```python
from build123d import *

# Parameters (mm, degrees)
F0_W     = 55
F0_H     = 14.5
F3_DEPTH = 55
F4_R     = 4
F5_DEPTH = 16.001
F7_DEPTH = 55
F4_R_2   = 6.5
F8_DEPTH = 6


with BuildPart() as f1:
    # F0 (on Front) → F1 (revolve)
    with BuildSketch(Plane.XZ):
        with Locations((-27.5, 7.25)):
            Rectangle(F0_W, F0_H)
        Polygon((0, 16), (0, 14.5), (0, 0), (25, 0), (25, 14.5), (5, 14.5), (5, 16), align=None)
    revolve(axis=Axis((-15, 0, 0), (-1, 0, 0)))

    # F2 (on face) → F3 (cut)
    with BuildSketch(Plane(origin=(-55, 0, 0), x_dir=(0, -1, 0), z_dir=(-1, 0, 0))):
        with BuildLine():
            ThreePointArc((14.5, 0), (0, 14.5), (-14.5, 0))
            Line((-14.5, 0), (14.5, 0))
        make_face()
    extrude(amount=-F3_DEPTH, mode=Mode.SUBTRACT)

    # F4 (on face) → F5 (cut, through all)
    with BuildSketch(Plane.XY):
        with Locations((-38, 0)):
            Circle(F4_R)
        with Locations((-18, 0)):
            Circle(F4_R)
    extrude(amount=-F5_DEPTH, mode=Mode.SUBTRACT)

    # F6 (on face) → F7 (cut)
    with BuildSketch(Plane(origin=(-55, 0, 0), x_dir=(0, -1, 0), z_dir=(-1, 0, 0))):
        with BuildLine():
            ThreePointArc((-5.546382, -13.3973), (0.699618, -14.483112), (6.811879, -12.800325))
            Line((6.811879, -12.800325), (6.811879, -11.710467))
            Line((6.811879, -11.710467), (-5.546382, -11.710467))
            Line((-5.546382, -11.710467), (-5.546382, -13.3973))
        make_face()
    extrude(amount=-F7_DEPTH, mode=Mode.SUBTRACT)

    # F4 (on face) → F8 (cut)
    with BuildSketch(Plane.XY):
        with Locations((-38, 0)):
            Circle(F4_R_2)
        with Locations((-38, 0)):
            Circle(F4_R, mode=Mode.SUBTRACT)
        with Locations((-18, 0)):
            Circle(F4_R_2)
        with Locations((-18, 0)):
            Circle(F4_R, mode=Mode.SUBTRACT)
    extrude(amount=-F8_DEPTH, mode=Mode.SUBTRACT)


solid = f1.part
```
The listing builds one solid part. Answer for the finished solid, in the listing's coordinates (mm). A direction names the side the tool comes from. Round coordinates to 2 decimals unless told otherwise and drop trailing zeros. Loops run counter-clockwise (first coordinate to the right, second up) from the corner with the lowest first, then second, coordinate; pieces in that order, holes last. Notation, with made-up numbers: (86.5, 36) -> (100.5, 36) arc R21 ccw to (100.5, 41) -> close; hole circle Ø8 at (44, 69). An arc over 180 degrees is marked (long way). Use one line per item in the form item = value.
1. The part is cut by section A-A on y = 0. Determine the outline of the cut face in (x, z), and give its area (3 significant figures).
Answer key:
outline = (-55, -11.71) -> (-42, -11.71) -> (-42, -6) -> (-44.5, -6) -> (-44.5, 0) -> (-55, 0) -> close; (-34, -11.71) -> (-22, -11.71) -> (-22, -6) -> (-24.5, -6) -> (-24.5, 0) -> (-31.5, 0) -> (-31.5, -6) -> (-34, -6) -> close; (-14, -11.71) -> (0, -11.71) -> (0, -16) -> (5, -16) -> (5, -14.5) -> (25, -14.5) -> (25, 14.5) -> (5, 14.5) -> (5, 16) -> (0, 16) -> (0, 0) -> (-11.5, 0) -> (-11.5, -6) -> (-14, -6) -> close
area = 1,140 mm²
2. For a pull along X with two mould halves and no side action, classify faces 5 (the cylindrical face through (14.86, -12.864, 6.691)), 6 (the cylindrical face through (-21.2, -2.4, -8.8)), 7 (the flat face through (25, 0, 0)) as released by +X, released by -X, zero draft, split by the parting line, or undercut.
Answer key:
face_5 = zero draft
face_6 = undercut
face_7 = released by +X
3. The part is cut by section D-D on y = -10. Determine the outline of the cut face in (x, z).
Answer key:
outline = (-55, -10.5) -> (0, -10.5) -> (0, -12.49) -> (5, -12.49) -> (5, -10.5) -> (25, -10.5) -> (25, 10.5) -> (5, 10.5) -> (5, 12.49) -> (0, 12.49) -> (0, 0) -> (-55, 0) -> close
4. The part is cut by section B-B on x = -38. Determine the outline of the cut face in (y, z), and give its area (3 significant figures).
Answer key:
outline = (-14.5, 0) arc R14.5 ccw to (-6.81, -12.8) -> (-6.81, -11.71) -> (-4, -11.71) -> (-4, -6) -> (-6.5, -6) -> (-6.5, 0) -> close; (4, -11.71) -> (5.55, -11.71) -> (5.55, -13.4) arc R14.5 ccw to (14.5, 0) -> (6.5, 0) -> (6.5, -6) -> (4, -6) -> close
area = 178 mm²
5. The part is cut by section C-C on z = -8.5. Determine the outline of the cut face in (x, y), and give its area (3 significant figures).
Answer key:
outline = (-55, -11.75) -> (0, -11.75) -> (0, -13.56) -> (5, -13.56) -> (5, -11.75) -> (25, -11.75) -> (25, 11.75) -> (5, 11.75) -> (5, 13.56) -> (0, 13.56) -> (0, 11.75) -> (-55, 11.75) -> close; hole circle Ø8 at (-38, 0); hole circle Ø8 at (-18, 0)
area = 1,800 mm²
6. Flat-ended cylindrical pins translate along their axes: pin 1 Ø4 at (x, y) = (-8, 4.5) entering from +Z; pin 2 Ø1.5 at (x, y) = (7, 5) entering from -Z; pin 3 Ø0.8 at (x, z) = (-29.5, -12) entering from -Y; pin 4 Ø7 at (x, y) = (-18, 0) entering from +Z. Find the tip coordinate at first contact, or state that the pin passes through.
Answer key:
pin_1 = 0
pin_2 = -13.86
pin_3 = -8.7
pin_4 = through
7. Find the intervals of material crossed by probe 1 along Z at (x, y) = (-4, 2); probe 2 along Y at (x, z) = (-51.5, -12.5); probe 3 along Y at (x, z) = (3.5, 0), in increasing order. Write a range as [from, to].
Answer key:
probe_1 = [-11.71, 0]
probe_2 = [-7.35, -6.81], [5.55, 7.35]
probe_3 = [-16, 16]
8. A tool of negligible diameter and unlimited length cuts with its end or side. For faces 1 (the cylindrical face through (-27.12, 12.12, -7.96)), 2 (the flat face through (-28, -1, -11.71)), 3 (the flat face through (-28, 0, 0)), 4 (the cylindrical face through (-24.494, 0.286, -2.958)), from which of +Z, -Z, +X, -X, +Y, -Y can it reach the whole face along a straight path? Write none if from no direction.
Answer key:
face_1 = -Z, -X, +Y
face_2 = -Z, -X
face_3 = +Z, -X, +Y, -Y
face_4 = +Z
